```python
from build123d import *

# Parameters (mm, degrees)
F1_DEPTH = 20
F3_DEPTH = 20
F5_DEPTH = 25
F7_DEPTH = 10


with BuildPart() as f1:
    # F0 (on Front) → F1 (new body)
    with BuildSketch(Plane.XZ):
        Polygon((-25, -10), (25, -10), (25, 10), (-10, 10), (-10, 80), (25, 80), (25, 90), (-10, 90), (-25, 90), (-25, 10), align=None)
    extrude(amount=F1_DEPTH)

    # F2 (on face) → F3 (cut)
    with BuildSketch(Plane.XY.offset(10)):
        Polygon((12.5, -12.5), (12.5, -7.5), (7.5, -7.5), (7.5, -12.5), (7.5, -20), (12.5, -20), align=None)
    extrude(amount=-F3_DEPTH, mode=Mode.SUBTRACT)

    # F4 (on face) → F5 (cut)
    with BuildSketch(Plane.XY.offset(90)):
        with BuildLine():
            ThreePointArc((9.8, -10.2), (10, -10.4), (10.2, -10.2))
            Line((10.2, -10.2), (10.2, -9.8))
            ThreePointArc((10.2, -9.8), (10, -9.6), (9.8, -9.8))
            Line((9.8, -9.8), (9.8, -10.2))
        make_face()
    extrude(amount=-F5_DEPTH, mode=Mode.SUBTRACT)

    # F6 (on face) → F7 (cut)
    with BuildSketch(Plane.XY.offset(90)):
        Polygon((25, -20), (25, -12), (10.40748, -12), (10.25, -10.2), (10.2, -10.2), (9.8, -10.2), (9.75, -10.2), (9.59252, -12), (-25, -12), (-25, -20), align=None)
    extrude(amount=-F7_DEPTH, mode=Mode.SUBTRACT)


solid = f1.part
```
Read the model definition and answer for the solid it produces. Units are mm, in the model's axes. A direction names the side the tool comes from. Coordinates: 2 decimals unless noted, no trailing zeros. Loops run counter-clockwise (first coordinate to the right, second up) from the corner with the lowest first, then second, coordinate; pieces in that order, holes last. Notation, with made-up numbers: (7.25, 19) - (65.25, 19) arc R28 ccw to (65.25, 40) - close; hole circle Ø11 at (-7, 8.5). An arc over 180 degrees is marked (long way). Answer in a Markdown table with one row per item.
1. Find section D-D, the plane y = -1.5. Write down the section's boundary in (x, z).
Conclusion:
| item | result |
|---|---|
| outline | (-25, -10) - (25, -10) - (25, 10) - (-10, 10) - (-10, 80) - (25, 80) - (25, 90) - (-25, 90) - close |
2. Straight lines are drawn through the part: line 1 (Z direction, x = 12.5, y = -1); line 2 (X direction, y = -9.5, z = 9); line 3 (Z direction, x = 7, y = -17.75). For each, find the intervals that lie inside material, in ascending order.
Conclusion:
| item | result |
|---|---|
| line 1 | z = -10 to 10, 80 to 90 |
| line 2 | x = -25 to 7.5, 12.5 to 25 |
| line 3 | z = -10 to 10 |
3. Determine the mould class of faces 5 (the face through (-16, -20, 26)), 6 (the face through (0, -6, 90)), 7 (the face through (-10, -10, 45)) for opening direction Z: +Z half, -Z half, draft (parallel to the pull), parting line (faces both ways), or undercut.
Conclusion:
| item | result |
|---|---|
| face 5 | draft |
| face 6 | +Z half |
| face 7 | undercut |
4. Find section C-C, the plane z = 2. Write down the section's boundary in (x, y), then the cut area to 4 significant figures.
Conclusion:
| item | result |
|---|---|
| outline | (-25, -20) - (7.5, -20) - (7.5, -7.5) - (12.5, -7.5) - (12.5, -20) - (25, -20) - (25, 0) - (-25, 0) - close |
| area | 937.5 mm² |
5. Find section B-B, the plane y = -8.5. Write down the section's boundary in (x, z).
Conclusion:
| item | result |
|---|---|
| outline | (-25, -10) - (7.5, -10) - (7.5, 10) - (-10, 10) - (-10, 80) - (25, 80) - (25, 90) - (-25, 90) - close; (12.5, -10) - (25, -10) - (25, 10) - (12.5, 10) - close |
6. Given pin 1 (3 mm diameter, centred on y = -12.5, z = 67.5, fed in from +X); pin 2 (11 mm diameter, centred on x = -13, z = 87.5, fed in from -Y); pin 3 (4 mm diameter, centred on x = -17, y = -17, fed in from +Z), each flat-ended and moving along its own axis, determine where each tip first touches the part or whether it passes through.
Conclusion:
| item | result |
|---|---|
| pin 1 | stops at x = -10 |
| pin 2 | stops at y = -12 |
| pin 3 | stops at z = 80 |
7. Which of the six approach directions +Z, -Z, +X, -X, +Y, -Y give full straight-line access (tool end or side, diameter ignored) to faces 1 (the face through (9.672, -11.087, 85.07)), 2 (the face through (-18, -16, 80)), 3 (the face through (4, -10, 10)), 4 (the face through (7.5, -14, 0))?
Conclusion:
| item | result |
|---|---|
| face 1 | +Z, -Z, -Y |
| face 2 | +Z, +X, -X, -Y |
| face 3 | +X, +Y, -Y |
| face 4 | -Z, -Y |
8. Find section A-A, the plane x = 16.5. Write down the section's boundary in (y, z), then the cut area to 3 significant figures.
Conclusion:
| item | result |
|---|---|
| outline | (-20, -10) - (0, -10) - (0, 10) - (-20, 10) - close; (-12, 80) - (0, 80) - (0, 90) - (-12, 90) - close |
| area | 520 mm² |
